For this review, take the finished solid that the model builds, in its own axes (mm). Coordinates: 2 decimals unless noted, no trailing zeros.
```python
from build123d import *

# Parameters (mm, degrees)
SKETCH1_R           = 2.5
BOSS_EXTRUDE1_DEPTH = 300


with BuildPart() as part:
    # Sketch1 → Boss-Extrude1 (new body)
    with BuildSketch(Plane(origin=(0, 0, 0), x_dir=(1, 0, 0), z_dir=(0, 1, 0))):
        with BuildLine():
            Line((-6.597918472, 7.658578644), (-2.997918472, 4.058578644))
            ThreePointArc((-2.997918472, 4.058578644), (-2.933033802, 4.015224093), (-2.856497116, 4))
            Line((-2.856497116, 4), (-0.211803399, 4))
            ThreePointArc((-0.211803399, 4), (-0.200315753, 3.998662449), (-0.189442719, 3.99472136))
            Line((-0.189442719, 3.99472136), (0, 3.9))
            Line((0, 3.9), (0.189442719, 3.99472136))
            ThreePointArc((0.189442719, 3.99472136), (0.200315753, 3.998662449), (0.211803399, 4))
            Line((0.211803399, 4), (2.856497116, 4))
            ThreePointArc((2.856497116, 4), (2.933033802, 4.015224093), (2.997918472, 4.058578644))
            Line((2.997918472, 4.058578644), (6.597918472, 7.658578644))
            ThreePointArc((6.597918472, 7.658578644), (6.641273022, 7.876536686), (6.456497116, 8))
            Line((6.456497116, 8), (3.2, 8))
            ThreePointArc((3.2, 8), (3.058578644, 8.058578644), (3, 8.2))
            Line((3, 8.2), (3, 9.8))
            ThreePointArc((3, 9.8), (3.058578644, 9.941421356), (3.2, 10))
            Line((3.2, 10), (9.8, 10))
            ThreePointArc((9.8, 10), (9.941421356, 9.941421356), (10, 9.8))
            Line((10, 9.8), (10, 3.2))
            ThreePointArc((10, 3.2), (9.941421356, 3.058578644), (9.8, 3))
            Line((9.8, 3), (8.2, 3))
            ThreePointArc((8.2, 3), (8.058578644, 3.058578644), (8, 3.2))
            Line((8, 3.2), (8, 6.456497116))
            ThreePointArc((8, 6.456497116), (7.876536686, 6.641273022), (7.658578644, 6.597918472))
            Line((7.658578644, 6.597918472), (4.058578644, 2.997918472))
            ThreePointArc((4.058578644, 2.997918472), (4.015224093, 2.933033802), (4, 2.856497116))
            Line((4, 2.856497116), (4, 0.130901699))
            ThreePointArc((4, 0.130901699), (3.99253254, 0.104615144), (3.97236068, 0.08618034))
            Line((3.97236068, 0.08618034), (3.8, 0))
            Line((3.8, 0), (3.97236068, -0.08618034))
            ThreePointArc((3.97236068, -0.08618034), (3.99253254, -0.104615144), (4, -0.130901699))
            Line((4, -0.130901699), (4, -2.856497116))
            ThreePointArc((4, -2.856497116), (4.015224093, -2.933033802), (4.058578644, -2.997918472))
            Line((4.058578644, -2.997918472), (7.658578644, -6.597918472))
            ThreePointArc((7.658578644, -6.597918472), (7.876536686, -6.641273022), (8, -6.456497116))
            Line((8, -6.456497116), (8, -3.2))
            ThreePointArc((8, -3.2), (8.058578644, -3.058578644), (8.2, -3))
            Line((8.2, -3), (9.8, -3))
            ThreePointArc((9.8, -3), (9.941421356, -3.058578644), (10, -3.2))
            Line((10, -3.2), (10, -9.8))
            ThreePointArc((10, -9.8), (9.941421356, -9.941421356), (9.8, -10))
            Line((9.8, -10), (3.2, -10))
            ThreePointArc((3.2, -10), (3.058578644, -9.941421356), (3, -9.8))
            Line((3, -9.8), (3, -8.2))
            ThreePointArc((3, -8.2), (3.058578644, -8.058578644), (3.2, -8))
            Line((3.2, -8), (6.456497116, -8))
            ThreePointArc((6.456497116, -8), (6.641273022, -7.876536686), (6.597918472, -7.658578644))
            Line((6.597918472, -7.658578644), (2.997918472, -4.058578644))
            ThreePointArc((2.997918472, -4.058578644), (2.933033802, -4.015224093), (2.856497116, -4))
            Line((2.856497116, -4), (0.211803399, -4))
            ThreePointArc((0.211803399, -4), (0.200315753, -3.998662449), (0.189442719, -3.99472136))
            Line((0.189442719, -3.99472136), (0, -3.9))
            Line((0, -3.9), (-0.189442719, -3.99472136))
            ThreePointArc((-0.189442719, -3.99472136), (-0.200315753, -3.998662449), (-0.211803399, -4))
            Line((-0.211803399, -4), (-2.856497116, -4))
            ThreePointArc((-2.856497116, -4), (-2.933033802, -4.015224093), (-2.997918472, -4.058578644))
            Line((-2.997918472, -4.058578644), (-6.597918472, -7.658578644))
            ThreePointArc((-6.597918472, -7.658578644), (-6.641273022, -7.876536686), (-6.456497116, -8))
            Line((-6.456497116, -8), (-3.2, -8))
            ThreePointArc((-3.2, -8), (-3.058578644, -8.058578644), (-3, -8.2))
            Line((-3, -8.2), (-3, -9.8))
            ThreePointArc((-3, -9.8), (-3.058578644, -9.941421356), (-3.2, -10))
            Line((-3.2, -10), (-9.8, -10))
            ThreePointArc((-9.8, -10), (-9.941421356, -9.941421356), (-10, -9.8))
            Line((-10, -9.8), (-10, -3.2))
            ThreePointArc((-10, -3.2), (-9.941421356, -3.058578644), (-9.8, -3))
            Line((-9.8, -3), (-8.2, -3))
            ThreePointArc((-8.2, -3), (-8.058578644, -3.058578644), (-8, -3.2))
            Line((-8, -3.2), (-8, -6.456497116))
            ThreePointArc((-8, -6.456497116), (-7.876536686, -6.641273022), (-7.658578644, -6.597918472))
            Line((-7.658578644, -6.597918472), (-4.058578644, -2.997918472))
            ThreePointArc((-4.058578644, -2.997918472), (-4.015224093, -2.933033802), (-4, -2.856497116))
            Line((-4, -2.856497116), (-4, -0.130901699))
            ThreePointArc((-4, -0.130901699), (-3.99253254, -0.104615144), (-3.97236068, -0.08618034))
            Line((-3.97236068, -0.08618034), (-3.8, 0))
            Line((-3.8, 0), (-3.97236068, 0.08618034))
            ThreePointArc((-3.97236068, 0.08618034), (-3.99253254, 0.104615144), (-4, 0.130901699))
            Line((-4, 0.130901699), (-4, 2.856497116))
            ThreePointArc((-4, 2.856497116), (-4.015224093, 2.933033802), (-4.058578644, 2.997918472))
            Line((-4.058578644, 2.997918472), (-7.658578644, 6.597918472))
            ThreePointArc((-7.658578644, 6.597918472), (-7.876536686, 6.641273022), (-8, 6.456497116))
            Line((-8, 6.456497116), (-8, 3.2))
            ThreePointArc((-8, 3.2), (-8.058578644, 3.058578644), (-8.2, 3))
            Line((-8.2, 3), (-9.8, 3))
            ThreePointArc((-9.8, 3), (-9.941421356, 3.058578644), (-10, 3.2))
            Line((-10, 3.2), (-10, 9.8))
            ThreePointArc((-10, 9.8), (-9.941421356, 9.941421356), (-9.8, 10))
            Line((-9.8, 10), (-3.2, 10))
            ThreePointArc((-3.2, 10), (-3.058578644, 9.941421356), (-3, 9.8))
            Line((-3, 9.8), (-3, 8.2))
            ThreePointArc((-3, 8.2), (-3.058578644, 8.058578644), (-3.2, 8))
            Line((-3.2, 8), (-6.456497116, 8))
            ThreePointArc((-6.456497116, 8), (-6.641273022, 7.876536686), (-6.597918472, 7.658578644))
        make_face()
        with Locations(Location((0, 0, 0), (0, 0, 270))):
            Circle(SKETCH1_R, mode=Mode.SUBTRACT)
    extrude(amount=BOSS_EXTRUDE1_DEPTH)


solid = part.part
```
1) Clearance check with flat-ended pins moving along their axes: P1, Ø0.8, axis at x = -1, y = 150.5, coming from the +Z side; P2, Ø3, axis at x = 1, y = 190, coming from the -Z side; P3, Ø1.4, axis at y = 170, z = -1, coming from the -X side. State where each tip first meets the part, or that it passes through.
2) The part is to be moulded in two halves that separate along X. For faces 1 (the face through (-2.44, 147.9, -0.54)), 2 (the face through (10, 148, 6)), 3 (the face through (-7, 148, -10)), say which applies: pulls with the +X half, pulls with the -X half, needs draft (parallel to the pull), parting line crosses it, or undercut.
3) For L1, parallel to X at y = 154, z = 0; L2, parallel to Z at x = 8.25, y = 178.5, list the stretches that pass through material, from the lowest coordinate up.
Results:
1. P1: stops at z = 4
1. P2: stops at z = -4
1. P3: stops at x = -4
2. face 1: undercut
2. face 2: pulls with the +X half
2. face 3: needs draft
3. L1: x = -3.8 to -2.5, 2.5 to 3.8
3. L2: z = -10 to -3, 3 to 10
